from build123d import *

# Parameters (mm, degrees)
SKETCH1_R           = 2.1
SKETCH1_R_2         = 7
BOSS_EXTRUDE1_DEPTH = 4
FILLET1_R           = 10
SKETCH2_R           = 3.9
CUT_EXTRUDE1_DEPTH  = 2.4
FILLET2_R           = 2


with BuildPart() as part:
    # Sketch1 → Boss-Extrude1 (new body)
    with BuildSketch(Plane(origin=(0, 0, 0), x_dir=(1, 0, 0), z_dir=(0, 1, 0))):
        with BuildLine():
            add(Edge.make_bspline(
                [(-48.276532762, 11.615114404), (-40.793059369, 8.635332343), (-34.627763453, 3.802891886), (-29.780645012, -2.882206965)],
                knots=[0.158174001, 0.158174001, 0.158174001, 0.158174001, 0.985694322, 0.985694322, 0.985694322, 0.985694322], degree=3))
            add(Edge.make_bspline(
                [(-29.780645012, -2.882206965), (-29.696850917, -2.997774969), (-29.613450765, -3.113896649), (-29.530444557, -3.230572003)],
                knots=[0.985694322, 0.985694322, 0.985694322, 0.985694322, 1, 1, 1, 1], degree=3))
            ThreePointArc((-29.530444557, -3.230572003), (-27.697474443, -4.713679973), (-25.4, -5.243774185))
            add(Edge.make_bspline(
                [(-25.4, -5.243774185), (-17.91803421, -6.039173757), (-10.43606842, -6.365978653)],
                knots=[0, 0, 0, 0.294565582, 0.294565582, 0.294565582], degree=2))
            ThreePointArc((-10.43606842, -6.365978653), (0, -12.224451247), (10.43606842, -6.365978653))
            add(Edge.make_bspline(
                [(10.43606842, -6.365978653), (17.918034209, -6.039173757), (25.4, -5.243774185)],
                knots=[0.705434418, 0.705434418, 0.705434418, 1, 1, 1], degree=2))
            ThreePointArc((25.4, -5.243774185), (29.107908285, -3.707908285), (30.643774185, 0))
            add(Edge.make_bspline(
                [(-46.474516908, 36.934762739), (-23.164206568, 39.351897946), (33.373901801, 38.120150773), (30.643774185, 0)],
                knots=[0, 0, 0, 0, 1, 1, 1, 1], degree=3))
            ThreePointArc((-46.474516908, 36.934762739), (-59.166363236, 25.114100216), (-48.276532762, 11.615114404))
        make_face()
        with Locations(Location((-25.4, 0, 0), (0, 0, 270))):
            Circle(SKETCH1_R, mode=Mode.SUBTRACT)
        with Locations(Location((0, 0, 0), (0, 0, 270))):
            Circle(SKETCH1_R_2, mode=Mode.SUBTRACT)
        with Locations(Location((25.4, 0, 0), (0, 0, 270))):
            Circle(SKETCH1_R, mode=Mode.SUBTRACT)
        with BuildLine():
            Line((6.818861244, 22.448276617), (14.692223791, 17.296643593))
            add(Edge.make_bspline(
                [(14.692223791, 17.296643593), (20.936611379, 11.517843997), (24.015411048, 1.179452343), (12.224451247, 0)],
                knots=[0.294731971, 0.294731971, 0.294731971, 0.294731971, 1, 1, 1, 1], degree=3))
            ThreePointArc((12.224451247, 0), (9.551728824, 7.629002869), (2.702275798, 11.922034801))
            Line((2.702275798, 11.922034801), (2.702275798, 18.575013303))
            ThreePointArc((2.702275798, 18.575013303), (5.139411914, 20.10900226), (6.818861244, 22.448276617))
        make_face(mode=Mode.SUBTRACT)
        with Locations(Location((-46.474516908, 24.210813251, 0), (0, 0, 270))):
            Circle(SKETCH1_R_2, mode=Mode.SUBTRACT)
        with BuildLine():
            add(Edge.make_bspline(
                [(-26.616347467, 28.001234406), (-23.355822424, 28.704578443), (-20.160458878, 28.867528343), (-17.03025683, 28.490084106)],
                knots=[0, 0, 0, 0, 0.490853217, 0.490853217, 0.490853217, 0.490853217], degree=3))
            add(Edge.make_bspline(
                [(-17.03025683, 28.490084106), (-16.127682529, 28.381250406), (-15.230525893, 28.227487183), (-14.338786924, 28.028794436)],
                knots=[0.490853217, 0.490853217, 0.490853217, 0.490853217, 0.632387691, 0.632387691, 0.632387691, 0.632387691], degree=3))
            Line((-14.338786924, 28.028794436), (-7.392215006, 26.83822498))
            ThreePointArc((-7.392215006, 26.83822498), (-6.522641563, 21.869230657), (-2.702275798, 18.575013303))
            Line((-2.702275798, 18.575013303), (-2.702275798, 11.922034801))
            ThreePointArc((-2.702275798, 11.922034801), (-9.215350555, 8.032093278), (-12.179376812, 1.048803495))
            Line((-12.179376812, 1.048803495), (-17.973694645, 1.048803495))
            ThreePointArc((-17.973694645, 1.048803495), (-21.967394814, 6.668374737), (-28.861522607, 6.653409745))
            Line((-28.861522607, 6.653409745), (-34.221790482, 12.01367762))
            add(Edge.make_bspline(
                [(-34.116347467, 20.501234406), (-35.2187538, 15.994576363), (-34.221790482, 12.01367762)],
                knots=[0, 0, 0, 0.526441047, 0.526441047, 0.526441047], degree=2))
            ThreePointArc((-34.116347467, 20.501234406), (-28.813046608, 22.697933547), (-26.616347467, 28.001234406))
        make_face(mode=Mode.SUBTRACT)
        with Locations(Location((-34.116347467, 28.001234406, 0), (0, 0, 270))):
            Circle(SKETCH1_R, mode=Mode.SUBTRACT)
        with Locations(Location((0, 25.57127698, 0), (0, 0, 270))):
            Circle(SKETCH1_R, mode=Mode.SUBTRACT)
    extrude(amount=BOSS_EXTRUDE1_DEPTH)

    # Fillet1
    fillet1_edges = [part.edges().sort_by_distance(p)[0] for p in [
        (10.43606842, 2, 6.365978653),
        (-10.43606842, 2, 6.365978653),
    ]]
    fillet(fillet1_edges, radius=FILLET1_R)

    # Sketch2 → Cut-Extrude1 (cut)
    with BuildSketch(Plane.XZ):
        with Locations(Location((0, -25.57127698, 0), (0, 0, 270))):
            Circle(SKETCH2_R)
        with Locations(Location((25.4, 0, 0), (0, 0, 270))):
            Circle(SKETCH2_R)
        with Locations(Location((-25.4, 0, 0), (0, 0, 270))):
            Circle(SKETCH2_R)
        with Locations(Location((-34.116347467, -28.001234406, 0), (0, 0, 270))):
            Circle(SKETCH2_R)
    extrude(amount=-CUT_EXTRUDE1_DEPTH, mode=Mode.SUBTRACT)

    # Fillet2
    fillet2_edges = [part.edges().sort_by_distance(p)[0] for p in [
        (-7.392215006, 2, -26.83822498),
        (-26.616347467, 2, -28.001234406),
        (-28.861522607, 2, -6.653409745),
        (-17.973694645, 2, -1.048803495),
        (12.224451247, 2, 0),
        (-34.116347467, 2, -20.501234406),
        (2.702275798, 2, -11.922034801),
        (2.702275798, 2, -18.575013303),
        (6.818861244, 2, -22.448276617),
        (-2.702275798, 2, -11.922034801),
        (-2.702275798, 2, -18.575013303),
    ]]
    fillet(fillet2_edges, radius=FILLET2_R)


solid = part.part
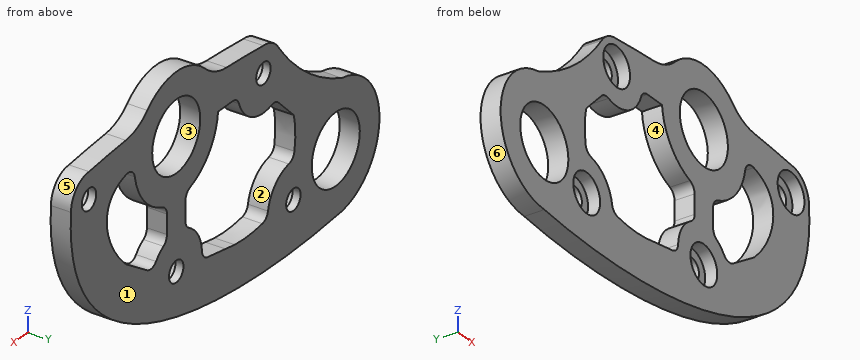
Source: CAD feature listing. Evaluate the final solid. Frame: model axes, mm. Face numbers are marked on the shaded views. A direction names the side the tool comes from. Coordinates: 2 decimals unless noted, no trailing zeros. One line per item, written item: value. Start each with the question number.
1. Mould query, pull axis X, two halves, no side actions, for the marked faces 3, 4, 5 and 6. Classes: pulls with the +X half, pulls with the -X half, needs draft (parallel to the pull), parting line crosses it, or undercut.
2. Ray query, L1, parallel to X at y = 2.95, z = -9; L2, parallel to Z at x = -25.4, y = 2.8; L3, parallel to X at y = 3.4, z = -6. Return the intervals inside material, ascending.
3. Section A-A (x = 0). State how many separate pieces and enclosed holes the cut face has, and give its area (3 significant figures).
4. Set-up query: the marked faces 1 and 2. Return all of +Z, -Z, +X, -X, +Y, -Y with unobstructed straight access to the full face (end or side cutting, diameter ignored); none if empty.
5. Contact query for flat-ended pins moving along their axis: P1, Ø1, axis at x = -40, y = 3.5, coming from the +Z side; P2, Ø6, axis at x = 0, z = -25.57, coming from the -Y side; P3, Ø1, axis at x = 18.5, y = 1.5, coming from the -Z side. Output: stop coordinate, or through.
Verdict:
1. face 3: undercut
1. face 4: undercut
1. face 5: pulls with the +X half
1. face 6: pulls with the -X half
2. L1: x = -42.85 to -31.21, -8.27 to 8.27, 19.93 to 30.1
2. L2: z = -37.59 to -28.22, -7.5 to -2.1, 2.1 to 5.24
2. L3: x = -38.35 to -20.9, -10.65 to -3.61, 3.61 to 10.65, 20.19 to 30.57
3. separate pieces: 3
3. enclosed holes: 0
3. area: 104 mm2
4. face 1: +Z, -Z, +X, -X, +Y
4. face 2: +Y, -Y
5. P1: stops at z = -6.85
5. P2: stops at y = 2.4
5. P3: stops at z = -26.41
